from build123d import *

# Parameters (mm, degrees)
EXTRUDE_1_DEPTH     = 3
SKETCH_2_W          = 3
SKETCH_2_H          = 0.95
CUT_EXTRUDE_1_DEPTH = 3
FILLET_1_R          = 1.27


with BuildPart() as part:
    # 스케치1 → 보스-돌출1 (new body)
    with BuildSketch(Plane.XY):
        with BuildLine():
            Line((-1.4475, 7.537196271), (1.4475, 7.537196271))
            Line((1.4475, 7.537196271), (1.4475, 4.537196271))
            ThreePointArc((1.4475, 4.537196271), (3.432437621, 3.301481217), (4.590044254, 1.27))
            ThreePointArc((4.590044254, 1.27), (10.408857131, 0), (4.590044254, -1.27))
            ThreePointArc((4.590044254, -1.27), (3.437893174, -3.295799869), (1.4625, -4.532383479))
            Line((1.4625, -4.532383479), (1.4625, -10.662668522))
            ThreePointArc((1.4625, -10.662668522), (3.822964303, -10.060633687), (5.987571718, -8.943175676))
            ThreePointArc((5.987571718, -8.943175676), (16.408857131, 0), (5.987571718, 8.943175676))
            ThreePointArc((5.987571718, 8.943175676), (0, 10.7625), (-5.987571718, 8.943175676))
            ThreePointArc((-5.987571718, 8.943175676), (-16.408857131, 0), (-5.987571718, -8.943175676))
            ThreePointArc((-5.987571718, -8.943175676), (-3.822964303, -10.060633687), (-1.4625, -10.662668522))
            Line((-1.4625, -10.662668522), (-1.4625, -4.532383479))
            ThreePointArc((-1.4625, -4.532383479), (-3.437893174, -3.295799869), (-4.590044254, -1.27))
            ThreePointArc((-4.590044254, -1.27), (-10.408857131, 0), (-4.590044254, 1.27))
            ThreePointArc((-4.590044254, 1.27), (-3.432437621, 3.301481217), (-1.4475, 4.537196271))
            Line((-1.4475, 4.537196271), (-1.4475, 7.537196271))
        make_face()
    extrude(amount=EXTRUDE_1_DEPTH)

    # 스케치2 → 컷-돌출1 (cut)
    with BuildSketch(Plane.XY.offset(3)):
        with Locations((14.908857131, -2.54)):
            Rectangle(SKETCH_2_W, SKETCH_2_H)
        with Locations((-14.908857131, -2.54)):
            Rectangle(SKETCH_2_W, SKETCH_2_H)
    extrude(amount=-CUT_EXTRUDE_1_DEPTH, mode=Mode.SUBTRACT)

    # 필렛1
    fillet_1_edges = [part.edges().sort_by_distance(p)[0] for p in [
        (-4.590044254, 1.27, 1.5),
        (-4.590044254, -1.27, 1.5),
        (-1.4625, -10.662668522, 1.5),
        (1.4625, -10.662668522, 1.5),
        (4.590044254, -1.27, 1.5),
        (4.590044254, 1.27, 1.5),
    ]]
    fillet(fillet_1_edges, radius=FILLET_1_R)


solid = part.part
Here's how the part is built. I have some questions about the finished solid (model axes, mm). A direction names the side the tool comes from. Round coordinates to 2 decimals unless told otherwise and drop trailing zeros. Order: outer loops, then holes, each group sorted by start corner. A loop starts at its lowest first (then second) coordinate and runs counter-clockwise, first axis right, second up. Notation, with made-up numbers: (-10, 23.5) -> (10, 23.5) arc R16 ccw to (10, 28.5) -> close; hole circle Ø8 at (68.5, 35.5). An arc over 180 degrees is marked (long way). Return JSON: item names as keys, results as strings.
Q1. If we mould it in two halves opening along X, with no side actions, what happens to faces 6 (the cylindrical face through (10.407, 0.093, 1.479)), 7 (the flat face through (15, -3.015, 2))? For each: released by +X, released by -X, zero draft, split by the parting line, or undercut.
Filled sheet:
{"face 6": "undercut", "face 7": "zero draft"}
Q2. If we section it at C-C on y = 8.25: List the corners of the cut face in (x, z) for me, plus the area to 3 significant figures.
Filled sheet:
{"outline": "(-11.08, 0) -> (11.08, 0) -> (11.08, 3) -> (-11.08, 3) -> close", "area": "66.5 mm^2"}
Q3. I need wall thicknesses on line 1 along Y through (x, z) = (-7.5, 2.65); line 2 along Y through (x, z) = (-3.5, 1.05); line 3 along Y through (x, z) = (0, 0.55). Which ranges of each line are inside material? Lowest first, please. Write a range as from..to.
Filled sheet:
{"line 1": "y = -9.05..-3.04, 3.04..9.05", "line 2": "y = -10.18..-3.23, 3.23..10.18", "line 3": "y = 7.54..10.76"}
Q4. For pin 1 Ø0.9 at (y, z) = (6, 1) entering from -X; pin 2 Ø1 at (y, z) = (2, 1) entering from +X; pin 3 Ø1.5 at (x, z) = (-8, 0.5) entering from -Y; pin 4 Ø3.5 at (x, y) = (-7.36, 0) entering from +Z, each with a flat end and sliding along its axis, tell me the tip position at first contact or that it passes through.
Filled sheet:
{"pin 1": "stops at x = -14.51", "pin 2": "stops at x = 16.28", "pin 3": "stops at y = -9.05", "pin 4": "passes through"}
Q5. If we section it at B-B on x = -14: List the corners of the cut face in (y, z) for me (3 decimals), plus the area to 3 significant figures.
Filled sheet:
{"outline": "(-6.147, 0) -> (-3.015, 0) -> (-3.015, 3) -> (-6.147, 3) -> close; (-2.065, 0) -> (6.147, 0) -> (6.147, 3) -> (-2.065, 3) -> close", "area": "34.0 mm^2"}
Q6. Which directions (+Z, -Z, +X, -X, +Y, -Y) give clear straight access to the entire face, cutting with the end or side of a thin tool? Please do faces 1 (the flat face through (-15, -2.065, 2)), 2 (the flat face through (-4, -4, 0)), 3 (the flat face through (-1.448, 6, 1)), 4 (the flat face through (15, -2.065, 2)), 5 (the cylindrical face through (2.775, 3.871, 1.479)).
Filled sheet:
{"face 1": "+Z, -Z, -X", "face 2": "-Z, +X, -X, +Y, -Y", "face 3": "+Z, -Z, -Y", "face 4": "+Z, -Z, +X", "face 5": "+Z, -Z"}
Q7. If we section it at A-A on y = 0: List the corners of the cut face in (x, z) for me, plus the area to 3 significant figures.
Filled sheet:
{"outline": "(-16.41, 0) -> (-10.41, 0) -> (-10.41, 3) -> (-16.41, 3) -> close; (10.41, 0) -> (16.41, 0) -> (16.41, 3) -> (10.41, 3) -> close", "area": "36.0 mm^2"}
